Here's how the part is built. I have some questions about the finished solid (model axes, mm). A direction names the side the tool comes from. Coordinates: 2 decimals unless noted, no trailing zeros. Loops run counter-clockwise (first coordinate to the right, second up) from the corner with the lowest first, then second, coordinate; pieces in that order, holes last. Notation, with made-up numbers: (62, 8.25) -> (101, 8.25) arc R11 ccw to (101, 21.25) -> close; hole circle Ø1 at (23, -1). An arc over 180 degrees is marked (long way). Answer as a JSON object with one key per item and string values. Group by question number.
1) I'm going to push flat-ended pins straight in: pin 1 (8 mm diameter, centred on x = 15.24, z = 447.04, fed in from +Y); pin 2 (11.5 mm diameter, centred on y = 12.7, z = 127, fed in from -X); pin 3 (14.5 mm diameter, centred on y = 12.7, z = 396.24, fed in from -X). Where does each tip first touch, or does it pass through?
2) I need wall thicknesses on probe 1 along X at (y, z) = (0.9, 243.84); probe 2 along X at (y, z) = (17.5, 179); probe 3 along Z at (x, y) = (15.24, 1.1). Which ranges of each line are inside material? Lowest first, please. Write a range as [from, to].
3) I want a section at A-A (z = 294.64). Write out the boundary of the cut face in (x, y).
4) I want a section at C-C (z = 394). Write out the boundary of the cut face in (x, y), then the cut area to 3 significant figures.
5) I want a section at B-B (y = 12.7). Count the separate pieces of the cut face and the enclosed holes in it, then the cut area to 3 significant figures.
6) Which directions (+Z, -Z, +X, -X, +Y, -Y) give clear straight access to the entire face, cutting with the end or side of a thin tool? Please do faces 1 (the flat face through (50.8, 13, 225)), 2 (the flat face through (25, 2.54, 225)).
7) If we mould it in two halves opening along Y, with no side actions, what happens to faces 3 (the flat face through (26, 0, 225)), 4 (the cylindrical face through (14.47, 1.25, 240.37)), 5 (the cylindrical face through (49.512, 10.268, 300.506))? For each: +Y half, -Y half, draft (parallel to the pull), parting line (faces both ways), or undercut.
```python
from build123d import *

# Parameters (mm, degrees)
BOSS_EXTRUDE1_DEPTH = 457.2
CUT_EXTRUDE1_REACH  = 27.4
SKETCH2_R           = 3.556
CUT_EXTRUDE2_REACH  = 27.4
SKETCH3_R           = 3.556
SKETCH4_R           = 6.35
CUT_EXTRUDE3_DEPTH  = 51.8


with BuildPart() as part:
    # Sketch1 → Boss-Extrude1 (new body)
    with BuildSketch(Plane.XY):
        Polygon((48.26, 2.54), (48.26, 25.4), (50.8, 25.4), (50.8, 0), (0, 0), (0, 25.4), (2.54, 25.4), (2.54, 2.54), align=None)
    extrude(amount=BOSS_EXTRUDE1_DEPTH)

    # Sketch2 → Cut-Extrude1 (cut, up to next)
    with BuildSketch(Plane.XZ, mode=Mode.PRIVATE) as cut_extrude1_sk1:
        with Locations((15.24, 447.04)):
            Circle(SKETCH2_R)
    cut_extrude1_tool1 = extrude(cut_extrude1_sk1.sketch, amount=-CUT_EXTRUDE1_REACH, mode=Mode.PRIVATE) & part.part
    add(cut_extrude1_tool1.solids().sort_by_distance((15.24, 0, 447.04))[0], mode=Mode.SUBTRACT)
    # Sketch2 → Cut-Extrude1 (cut, up to next)
    with BuildSketch(Plane.XZ, mode=Mode.PRIVATE) as cut_extrude1_sk2:
        with Locations((35.56, 447.04)):
            Circle(SKETCH2_R)
    cut_extrude1_tool2 = extrude(cut_extrude1_sk2.sketch, amount=-CUT_EXTRUDE1_REACH, mode=Mode.PRIVATE) & part.part
    add(cut_extrude1_tool2.solids().sort_by_distance((35.56, 0, 447.04))[0], mode=Mode.SUBTRACT)

    # Sketch3 → Cut-Extrude2 (cut, up to next)
    with BuildSketch(Plane.XZ, mode=Mode.PRIVATE) as cut_extrude2_sk1:
        with Locations((15.24, 243.84)):
            Circle(SKETCH3_R)
    cut_extrude2_tool1 = extrude(cut_extrude2_sk1.sketch, amount=-CUT_EXTRUDE2_REACH, mode=Mode.PRIVATE) & part.part
    add(cut_extrude2_tool1.solids().sort_by_distance((15.24, 0, 243.84))[0], mode=Mode.SUBTRACT)
    # Sketch3 → Cut-Extrude2 (cut, up to next)
    with BuildSketch(Plane.XZ, mode=Mode.PRIVATE) as cut_extrude2_sk2:
        with Locations((35.56, 243.84)):
            Circle(SKETCH3_R)
    cut_extrude2_tool2 = extrude(cut_extrude2_sk2.sketch, amount=-CUT_EXTRUDE2_REACH, mode=Mode.PRIVATE) & part.part
    add(cut_extrude2_tool2.solids().sort_by_distance((35.56, 0, 243.84))[0], mode=Mode.SUBTRACT)

    # Sketch4 → Cut-Extrude3 (cut, through all)
    with BuildSketch(Plane.ZY):
        with Locations((396.24, 12.7)):
            Circle(SKETCH4_R)
        with Locations((294.64, 12.7)):
            Circle(SKETCH4_R)
        with Locations((127, 12.7)):
            Circle(SKETCH4_R)
    extrude(amount=-CUT_EXTRUDE3_DEPTH, mode=Mode.SUBTRACT)


solid = part.part
```
Determined:
{
 "1": {"pin 1": "y = 2.54", "pin 2": "through", "pin 3": "x = 0"},
 "2": {"probe 1": "[0, 11.68], [18.8, 32], [39.12, 50.8]", "probe 2": "[0, 2.54], [48.26, 50.8]", "probe 3": "[0, 240.28], [247.4, 443.48], [450.6, 457.2]"},
 "3": {"outline": "(0, 0) -> (50.8, 0) -> (50.8, 6.35) -> (48.26, 6.35) -> (48.26, 2.54) -> (2.54, 2.54) -> (2.54, 6.35) -> (0, 6.35) -> close; (0, 19.05) -> (2.54, 19.05) -> (2.54, 25.4) -> (0, 25.4) -> close; (48.26, 19.05) -> (50.8, 19.05) -> (50.8, 25.4) -> (48.26, 25.4) -> close"},
 "4": {"outline": "(0, 0) -> (50.8, 0) -> (50.8, 6.76) -> (48.26, 6.76) -> (48.26, 2.54) -> (2.54, 2.54) -> (2.54, 6.76) -> (0, 6.76) -> close; (0, 18.64) -> (2.54, 18.64) -> (2.54, 25.4) -> (0, 25.4) -> close; (48.26, 18.64) -> (50.8, 18.64) -> (50.8, 25.4) -> (48.26, 25.4) -> close", "area": "185 mm^2"},
 "5": {"separate pieces": "8", "enclosed holes": "0", "area": "2,130 mm^2"},
 "6": {"face 1": "+Z, -Z, +X, +Y, -Y", "face 2": "+Z, -Z, +Y"},
 "7": {"face 3": "-Y half", "face 4": "draft", "face 5": "undercut"}
}
